For this review, use the dimensioned drawing (mm, ordinates from the lowest corner) and the shaded views. Round coordinates to 2 decimals unless told otherwise and drop trailing zeros. Loops run counter-clockwise (first coordinate to the right, second up) from the corner with the lowest first, then second, coordinate; pieces in that order, holes last. Notation, with made-up numbers: M 0.25,-29.5 L 23.25,-29.5 A13 ccw 23.25,-25.5 Z; hole C 84.5,-37.5 d2. An arc over 180 degrees is marked long. Answer as a JSON object with one key per item and string values. Group by question number.
Item 1: Consider section A-A (x = 77.5). Give the boundary of the cut face in (y, z) (1 decimal).
Item 2: Consider section B-B (z = 2.3). Give the boundary of the cut face in (x, y) (1 decimal).
Item 3: Consider section C-C (y = 32.5). Give the boundary of the cut face in (x, z) (1 decimal).
Item 4: Consider section D-D (x = 65). Give the boundary of the cut face in (y, z).
Item 5: To check wall thickness, follow line 1 (Y direction, x = 77, z = 3.7) (1 decimal); line 2 (Y direction, x = 61.5, z = 5.15); line 3 (X direction, y = 37, z = 3.9) (1 decimal). State the ranges of each line that lie inside material, in increasing order.
Item 6: Insertion check: P1, Ø1.5, axis at y = 40.5, z = 4, coming from the +X side; P2, Ø3, axis at y = 30.5, z = 3.5, coming from the -X side; P3, Ø2.5, axis at x = 62.5, z = 2.5, coming from the +Y side. Each pin has a flat end and moves straight along its axis. Give the tip position at first contact, or say it passes through.
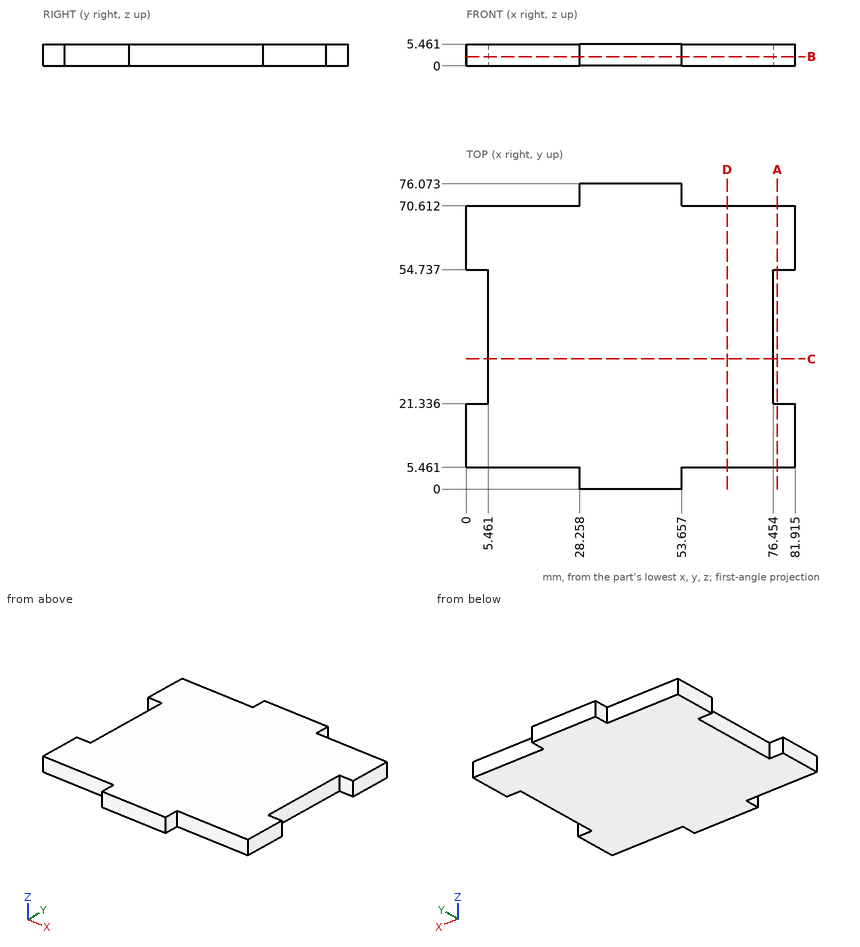
Geometry results:
{
 "1": {"outline": "M 5.5,0 L 21.3,0 L 21.3,5.5 L 5.5,5.5 Z; M 54.7,0 L 70.6,0 L 70.6,5.5 L 54.7,5.5 Z"},
 "2": {"outline": "M 0,5.5 L 28.3,5.5 L 28.3,0 L 53.7,0 L 53.7,5.5 L 81.9,5.5 L 81.9,21.3 L 76.5,21.3 L 76.5,54.7 L 81.9,54.7 L 81.9,70.6 L 53.7,70.6 L 53.7,76.1 L 28.3,76.1 L 28.3,70.6 L 0,70.6 L 0,54.7 L 5.5,54.7 L 5.5,21.3 L 0,21.3 Z"},
 "3": {"outline": "M 5.5,0 L 76.5,0 L 76.5,5.5 L 5.5,5.5 Z"},
 "4": {"outline": "M 5.46,0 L 70.61,0 L 70.61,5.46 L 5.46,5.46 Z"},
 "5": {"line 1": "y = 5.5 to 21.3, 54.7 to 70.6", "line 2": "y = 5.46 to 70.61", "line 3": "x = 5.5 to 76.5"},
 "6": {"P1": "stops at x = 76.45", "P2": "stops at x = 5.46", "P3": "stops at y = 70.61"}
}
